from build123d import *

# Parameters (mm, degrees)
SKETCH1_R           = 1.5875
BOSS_EXTRUDE2_DEPTH = 1.524


with BuildPart() as part:
    # Sketch1 → Boss-Extrude2 (new body)
    with BuildSketch(Plane(origin=(0, 0, 0), x_dir=(1, 0, 0), z_dir=(0, 1, 0))):
        with BuildLine():
            Line((-50.746188486, 35.427401309), (-17.726188486, 35.427401309))
            ThreePointArc((-17.726188486, 35.427401309), (-16.828162874, 35.055426921), (-16.456188486, 34.157401309))
            Line((-16.456188486, 34.157401309), (-16.456188486, 27.108901309))
            Line((-16.456188486, 27.108901309), (-16.456188486, 8.185901309))
            Line((-16.456188486, 8.185901309), (-16.456188486, 1.137401309))
            ThreePointArc((-16.456188486, 1.137401309), (-16.828162874, 0.239375697), (-17.726188486, -0.132598691))
            Line((-17.726188486, -0.132598691), (-50.746188486, -0.132598691))
            ThreePointArc((-50.746188486, -0.132598691), (-51.644214098, 0.239375697), (-52.016188486, 1.137401309))
            Line((-52.016188486, 1.137401309), (-52.016188486, 34.157401309))
            ThreePointArc((-52.016188486, 34.157401309), (-51.644214098, 35.055426921), (-50.746188486, 35.427401309))
        make_face()
        with Locations(Location((-49.539688486, 32.900101309, 0), (0, 0, 90))):
            Circle(SKETCH1_R, mode=Mode.SUBTRACT)
        with Locations(Location((-18.907288486, 32.900101309, 0), (0, 0, 90))):
            Circle(SKETCH1_R, mode=Mode.SUBTRACT)
        with Locations(Location((-18.907288486, 2.394701309, 0), (0, 0, 90))):
            Circle(SKETCH1_R, mode=Mode.SUBTRACT)
        with Locations(Location((-49.539688486, 2.394701309, 0), (0, 0, 90))):
            Circle(SKETCH1_R, mode=Mode.SUBTRACT)
    extrude(amount=BOSS_EXTRUDE2_DEPTH)


solid = part.part
The listing builds one solid part. Answer for the finished solid, in the listing's coordinates (mm). Give positions to 0.01 mm unless a question says otherwise; leave off trailing zeros. Order: outer loops, then holes, each group sorted by start corner. A loop starts at its lowest first (then second) coordinate and runs counter-clockwise, first axis right, second up. Notation, with made-up numbers: (14, 80.25) - (64, 80.25) arc R30 cw to (64, 103.25) - close; hole circle Ø9 at (81, 38.5). An arc over 180 degrees is marked (long way). One line per item, written item: value. Start each with the question number.
1) A cutting plane is placed at A-A on y = 0.95. Give the vertices of the cut face in (x, z) (1 decimal).
2) Find the intervals of material crossed by L1, parallel to Z at x = -20, y = 1.4; L2, parallel to X at y = 0.85, z = -2, in increasing order.
3) A cutting plane is placed at C-C on x = -49. Give the vertices of the cut face in (y, z), then the cut area to 3 significant figures.
4) Given pin 1 Ø3.5 at (x, z) = (-49.54, -2.39) entering from -Y, flat-ended and moving along its own axis, determine where the tip first touches the part or whether it passes through.
5) A cutting plane is placed at B-B on z = -3.5. Give the vertices of the cut face in (x, y).
6) The mould has two halves that part along Z. Classify faces 1 (the face through (-51.65, 0.75, -35.05)), 2 (the face through (-50.61, 0.75, -31.73)), 3 (the face through (-52.016, 1, -17)): released by +Z, released by -Z, zero draft, split by the parting line, or undercut.
Answer sheet:
1. outline: (-52, -34.2) arc R1.3 ccw to (-50.7, -35.4) - (-17.7, -35.4) arc R1.3 ccw to (-16.5, -34.2) - (-16.5, -1.1) arc R1.3 ccw to (-17.7, 0.1) - (-50.7, 0.1) arc R1.3 ccw to (-52, -1.1) - close; hole circle Ø3.2 at (-49.5, -32.9); hole circle Ø3.2 at (-49.5, -2.4); hole circle Ø3.2 at (-18.9, -32.9); hole circle Ø3.2 at (-18.9, -2.4)
2. L1: z = -35.43 to -34.05, -31.75 to -3.55, -1.24 to 0.13
2. L2: x = -52.02 to -51.08, -48 to -20.44, -17.37 to -16.46
3. outline: (0, -35.43) - (1.52, -35.43) - (1.52, -34.39) - (0, -34.39) - close; (0, -31.41) - (1.52, -31.41) - (1.52, -3.89) - (0, -3.89) - close; (0, -0.9) - (1.52, -0.9) - (1.52, 0.13) - (0, 0.13) - close
3. area: 45.1 mm2
4. pin 1: stops at y = 0
5. outline: (-52.02, 0) - (-50.68, 0) - (-50.68, 1.52) - (-52.02, 1.52) - close; (-48.4, 0) - (-20.05, 0) - (-20.05, 1.52) - (-48.4, 1.52) - close; (-17.77, 0) - (-16.46, 0) - (-16.46, 1.52) - (-17.77, 1.52) - close
6. face 1: released by -Z
6. face 2: undercut
6. face 3: zero draft
